CAD build for the part. Positions are in the model's coordinates, mm. A direction names the side the tool comes from. Give positions to 0.01 mm unless a question says otherwise; leave off trailing zeros. Loops run counter-clockwise (first coordinate to the right, second up) from the corner with the lowest first, then second, coordinate; pieces in that order, holes last.
Item 1: Drop flat-ended pins along their axis: P1, Ø1, axis at x = 6.5, z = 855.5, coming from the +Y side; P2, Ø10, axis at x = -25, z = 141.5, coming from the +Y side; P3, Ø3, axis at x = 19, y = 5.5, coming from the +Z side. Give the stop position or say it passes through.
Item 2: Mould opens along Y. For faces 1 (the flat face through (17.43, -17.925, 616.25)), 2 (the flat face through (0, 8, 1.25)), 3 (the flat face through (-18, 16, 1250)) say: released by +Y, released by -Y, zero draft, split by the parting line, or undercut.
Item 3: Which spindle directions (+Z, -Z, +X, -X, +Y, -Y) get a long thin tool onto all of the face, cutting with end or side? Do faces 4 (the flat face through (0, 8, 0)), 5 (the flat face through (16.56, -17.03, 616.88)). Say none if no direction does.
Item 4: Saw through at C-C on x = 21.5. Give the cut face in (y, z).
Item 5: Saw through at B-B on y = -20.5. Give the cut face in (x, z).
Item 6: Saw through at A-A on z = 235. Give the cut face in (x, y), plus the area to 3 significant figures.
Item 7: Probe probe 1 along Y at (x, z) = (0, 0.8); probe 2 along Z at (x, y) = (0, 8). List the from-to ranges inside material, lowest first.
from build123d import *

# Parameters (mm, degrees)
F1_DEPTH = 1250
F2_T     = -1.25
F3_R     = 4
F4_DEPTH = 12.5


with BuildPart() as f1:
    # F0 (on Top) → F1 (new body)
    with BuildSketch(Plane.XY):
        Polygon((35.355339, 0), (0, 35.355339), (-35.355339, 0), (0, -35.355339), align=None)
    extrude(amount=F1_DEPTH)

    # F2
    f2_openings = [f1.faces().sort_by_distance(p)[0] for p in [
        (0, 0, 1250),
    ]]
    offset(amount=F2_T, openings=f2_openings)

    # F3 (on face) → F4 (cut, symmetric)
    with BuildSketch(Plane(origin=(0, 0, 0), x_dir=(1, 0, 0), z_dir=(0, 0, -1))):
        Circle(F3_R)
    extrude(amount=F4_DEPTH, both=True, mode=Mode.SUBTRACT)


solid = f1.part
Results below:
1. P1: stops at y = 29.36
1. P2: stops at y = 15.36
1. P3: stops at z = 1.25
2. face 1: released by -Y
2. face 2: undercut
2. face 3: zero draft
3. face 4: -Z, +X, -X, +Y, -Y
3. face 5: +Z
4. outline: (-13.86, 0) - (13.86, 0) - (13.86, 1250) - (12.09, 1250) - (12.09, 1.25) - (-12.09, 1.25) - (-12.09, 1250) - (-13.86, 1250) - close
5. outline: (-14.86, 0) - (14.86, 0) - (14.86, 1250) - (13.09, 1250) - (13.09, 1.25) - (-13.09, 1.25) - (-13.09, 1250) - (-14.86, 1250) - close
6. outline: (-35.36, 0) - (0, -35.36) - (35.36, 0) - (0, 35.36) - close; hole (-33.59, 0) - (0, -33.59) - (33.59, 0) - (0, 33.59) - close
6. area: 244 mm2
7. probe 1: y = -35.36 to -4, 4 to 35.36
7. probe 2: z = 0 to 1.25
